```python
from build123d import *

# Parameters (mm, degrees)
F0_W     = 33
F0_H     = 5
F0_W_2   = 5
F0_H_2   = 33
F0_R     = 3
F1_DEPTH = 2
F2_DEPTH = 20
F0_R_2   = 1.522733
F3_DEPTH = 10


with BuildPart() as f1:
    # F0 (on Top) → F1 (new body)
    with BuildSketch(Plane.XY):
        with Locations((1.472682, 18.798609)):
            Rectangle(F0_W, F0_H)
        with Locations((-20.277318, -2.951391)):
            Rectangle(F0_W_2, F0_H_2)
        with BuildLine():
            Line((17.972682, 16.298609), (-15.027318, 16.298609))
            ThreePointArc((-15.027318, 16.298609), (-16.971862, 15.493153), (-17.777318, 13.548609))
            Line((-17.777318, 13.548609), (-17.777318, -19.451391))
            ThreePointArc((-17.777318, -19.451391), (-16.971862, -21.395934), (-15.027318, -22.201391))
            Line((-15.027318, -22.201391), (17.972682, -22.201391))
            ThreePointArc((17.972682, -22.201391), (19.917226, -21.395934), (20.722682, -19.451391))
            Line((20.722682, -19.451391), (20.722682, 13.548609))
            ThreePointArc((20.722682, 13.548609), (19.917226, 15.493153), (17.972682, 16.298609))
        make_face()
        with Locations((-13.777318, -18.201391)):
            Circle(F0_R, mode=Mode.SUBTRACT)
        with Locations((16.722682, -18.201391)):
            Circle(F0_R, mode=Mode.SUBTRACT)
        with Locations((-13.777318, 12.298609)):
            Circle(F0_R, mode=Mode.SUBTRACT)
        with Locations((16.722682, 12.298609)):
            Circle(F0_R, mode=Mode.SUBTRACT)
        with Locations((23.222682, -2.951391)):
            Rectangle(F0_W_2, F0_H_2)
        with Locations((1.472682, -24.701391)):
            Rectangle(F0_W, F0_H)
    extrude(amount=F1_DEPTH)

    # F0 (on Top) → F2 (join)
    with BuildSketch(Plane.XY):
        with BuildLine():
            ThreePointArc((-17.777318, 13.548609), (-16.971862, 15.493153), (-15.027318, 16.298609))
            Line((-15.027318, 16.298609), (-15.027318, 21.298609))
            ThreePointArc((-15.027318, 21.298609), (-20.507395, 19.028687), (-22.777318, 13.548609))
            Line((-22.777318, 13.548609), (-17.777318, 13.548609))
        make_face()
        with BuildLine():
            Line((17.972682, 21.298609), (17.972682, 16.298609))
            ThreePointArc((17.972682, 16.298609), (19.917226, 15.493153), (20.722682, 13.548609))
            Line((20.722682, 13.548609), (25.722682, 13.548609))
            ThreePointArc((25.722682, 13.548609), (23.45276, 19.028687), (17.972682, 21.298609))
        make_face()
        with BuildLine():
            Line((25.722682, -19.451391), (20.722682, -19.451391))
            ThreePointArc((20.722682, -19.451391), (19.917226, -21.395934), (17.972682, -22.201391))
            Line((17.972682, -22.201391), (17.972682, -27.201391))
            ThreePointArc((17.972682, -27.201391), (23.45276, -24.931468), (25.722682, -19.451391))
        make_face()
        with BuildLine():
            ThreePointArc((-15.027318, -22.201391), (-16.971862, -21.395934), (-17.777318, -19.451391))
            Line((-17.777318, -19.451391), (-22.777318, -19.451391))
            ThreePointArc((-22.777318, -19.451391), (-20.507395, -24.931468), (-15.027318, -27.201391))
            Line((-15.027318, -27.201391), (-15.027318, -22.201391))
        make_face()
    extrude(amount=F2_DEPTH)

    # F0 (on Top) → F3 (join)
    with BuildSketch(Plane.XY):
        with Locations((-13.777318, 12.298609)):
            Circle(F0_R)
        with Locations((-13.777318, 12.298609)):
            Circle(F0_R_2, mode=Mode.SUBTRACT)
        with Locations((16.722682, 12.298609)):
            Circle(F0_R)
        with Locations((16.722682, 12.298609)):
            Circle(F0_R_2, mode=Mode.SUBTRACT)
        with Locations((16.722682, -18.201391)):
            Circle(F0_R)
        with Locations((16.722682, -18.201391)):
            Circle(F0_R_2, mode=Mode.SUBTRACT)
        with Locations((-13.777318, -18.201391)):
            Circle(F0_R)
        with Locations((-13.777318, -18.201391)):
            Circle(F0_R_2, mode=Mode.SUBTRACT)
    extrude(amount=F3_DEPTH)


solid = f1.part
```
Model file for the job. Use its own axes, mm. A direction names the side the tool comes from. Round coordinates to 2 decimals unless told otherwise and drop trailing zeros. Write each loop counter-clockwise with the first axis right and the second up, starting at its lowest first coordinate (ties: lowest second). Pieces come first, ordered by that corner, then holes. Notation, with made-up numbers: M 63.5,36.5 L 116.5,36.5 A24 ccw 116.5,60.5 Z; hole C 18,51 d3. An arc over 180 degrees is marked long. Put each result on its own line as item: value.
Item 1: Cut at C-C (x = 22). List the corners of the cut face in (y, z), and give its area (3 significant figures).
Responses:
outline: M -26.07,0 L 20.17,0 L 20.17,20 L 13.55,20 L 13.55,2 L -19.45,2 L -19.45,20 L -26.07,20 Z
area: 331 mm²
Item 2: Cut at D-D (y = 18). List the corners of the cut face in (x, z).
Responses:
outline: M -21.37,0 L 24.32,0 L 24.32,20 L 17.97,20 L 17.97,2 L -15.03,2 L -15.03,20 L -21.37,20 Z
Item 3: Mould opens along X. For faces 4 (the cylindrical face through (-20.57, -24.87, 9.86)), 5 (the cylindrical face through (23.51, 18.97, 9.86)), 6 (the flat face through (23, -19.451, 11)), 7 (the cylindrical face through (19.938, -21.374, 10.874)) say: +X half, -X half, draft (parallel to the pull), parting line (faces both ways), or undercut.
Responses:
face 4: -X half
face 5: +X half
face 6: draft
face 7: undercut
Item 4: Cut at B-B (z = 6). State how many separate pieces and enclosed holes the cut face has, and give its area (3 significant figures).
Responses:
separate pieces: 8
enclosed holes: 4
area: 249 mm²
Item 5: Flat gauge pins, fed straight in: P1, Ø4, axis at y = -25.5, z = 13, coming from the +X side; P2, Ø5.5, axis at y = 18.5, z = 8.5, coming from the -X side; P3, Ø1.5, axis at x = 24, z = 13, coming from the +Y side; P4, Ø5, axis at x = -13.78, y = 12.3, coming from the -Z side. Where does each tip first touch, or does it go through?
Responses:
P1: x = 24.58
P2: x = -22.46
P3: y = 19.22
P4: z = 0
Item 6: Probe L1, parallel to Y at x = 17, z = 9; L2, parallel to Z at x = -5, y = 11; L3, parallel to Y at x = 20.5, z = 6. List the from-to ranges inside material, lowest first. Write a range as from..to.
Responses:
L1: -21.19..-19.7, -16.7..-15.21, 9.31..10.8, 13.8..15.29
L2: 0..2
L3: -26.78..-20.54, 14.63..20.87
Item 7: Cut at A-A (z = 11.5). List the corners of the cut face in (x, y).
Responses:
outline: M -22.78,-19.45 A7.75 ccw -15.03,-27.2 L -15.03,-22.2 A2.75 cw -17.78,-19.45 Z; M -22.78,13.55 L -17.78,13.55 A2.75 cw -15.03,16.3 L -15.03,21.3 A7.75 ccw Z; M 17.97,-27.2 A7.75 ccw 25.72,-19.45 L 20.72,-19.45 A2.75 cw 17.97,-22.2 Z; M 17.97,16.3 A2.75 cw 20.72,13.55 L 25.72,13.55 A7.75 ccw 17.97,21.3 Z
Item 8: Tool access for faces 1 (the cylindrical face through (15.2, -18.13, 4.93)), 2 (the flat face through (17.973, 19, 11)), 3 (the cylindrical face through (16.332, -15.227, 5.944)): list every direction of +Z, -Z, +X, -X, +Y, -Y with a clear straight run to the whole face (end or side of a thin tool).
Responses:
face 1: +Z, -Z
face 2: +Z, +Y
face 3: +Z
